CAD build for the part. Positions are in the model's coordinates, mm. Face numbers are marked on the shaded views. A direction names the side the tool comes from. Round coordinates to 2 decimals unless told otherwise and drop trailing zeros. Loops run counter-clockwise (first coordinate to the right, second up) from the corner with the lowest first, then second, coordinate; pieces in that order, holes last.
```python
from build123d import *

# Parameters (mm, degrees)
SKETCH1_W           = 86.36
SKETCH1_H           = 71.374
BOSS_EXTRUDE1_DEPTH = 39.624
FILLET1_R           = 2.54
CUT_EXTRUDE1_DEPTH  = 25.4
FILLET2_R           = 1.27
SKETCH4_W           = 49.53
SKETCH4_H           = 15.24
CUT_EXTRUDE2_DEPTH  = 50.8
SKETCH5_R           = 11.6205
BOSS_EXTRUDE2_DEPTH = 15.494
CUT_REVOLVE1_ANGLE  = 356


with BuildPart() as part:
    # Sketch1 → Boss-Extrude1 (new body)
    with BuildSketch(Plane(origin=(0, 0, 0), x_dir=(1, 0, 0), z_dir=(0, 1, 0))):
        with Locations((43.18, -35.687)):
            Rectangle(SKETCH1_W, SKETCH1_H)
    extrude(amount=BOSS_EXTRUDE1_DEPTH)

    # Fillet1
    fillet1_edges = [part.edges().sort_by_distance(p)[0] for p in [
        (0, 19.812, 0),
        (86.36, 19.812, 0),
        (86.36, 19.812, 71.374),
        (0, 19.812, 71.374),
    ]]
    fillet(fillet1_edges, radius=FILLET1_R)

    # Sketch2 → Cut-Extrude1 (cut)
    with BuildSketch(Plane.ZY):
        with BuildLine():
            Line((30.226, 33.02), (30.48, 33.02))
            ThreePointArc((30.48, 33.02), (31.737235857, 32.499235857), (32.258, 31.242))
            Line((32.258, 31.242), (32.258, 24.892))
            ThreePointArc((32.258, 24.892), (31.737235857, 23.634764143), (30.48, 23.114))
            Line((30.48, 23.114), (30.226, 23.114))
            ThreePointArc((30.226, 23.114), (28.968764143, 23.634764143), (28.448, 24.892))
            Line((28.448, 24.892), (28.448, 31.242))
            ThreePointArc((28.448, 31.242), (28.968764143, 32.499235857), (30.226, 33.02))
        make_face()
        with BuildLine():
            Line((41.148, 23.114), (40.894, 23.114))
            ThreePointArc((40.894, 23.114), (39.636764143, 23.634764143), (39.116, 24.892))
            Line((39.116, 24.892), (39.116, 31.242))
            ThreePointArc((39.116, 31.242), (39.636764143, 32.499235857), (40.894, 33.02))
            Line((40.894, 33.02), (41.148, 33.02))
            ThreePointArc((41.148, 33.02), (42.405235857, 32.499235857), (42.926, 31.242))
            Line((42.926, 31.242), (42.926, 24.892))
            ThreePointArc((42.926, 24.892), (42.405235857, 23.634764143), (41.148, 23.114))
        make_face()
    extrude(amount=-CUT_EXTRUDE1_DEPTH, mode=Mode.SUBTRACT)

    # Fillet2
    fillet2_edges = [part.edges().sort_by_distance(p)[0] for p in [
        (0, 23.634764143, 28.968764143),
        (0, 23.114, 30.353),
        (0, 23.634764143, 31.737235857),
        (0, 28.067, 32.258),
        (0, 32.499235857, 31.737235857),
        (0, 33.02, 30.353),
        (0, 32.499235857, 28.968764143),
        (0, 28.067, 28.448),
        (0, 23.634764143, 42.405235857),
        (0, 28.067, 42.926),
        (0, 32.499235857, 42.405235857),
        (0, 33.02, 41.021),
        (0, 32.499235857, 39.636764143),
        (0, 28.067, 39.116),
        (0, 23.634764143, 39.636764143),
        (0, 23.114, 41.021),
    ]]
    fillet(fillet2_edges, radius=FILLET2_R)

    # Sketch4 → Cut-Extrude2 (cut)
    with BuildSketch(Plane(origin=(86.36, 0, 0), x_dir=(0, 0, -1), z_dir=(1, 0, 0))):
        with Locations((-35.687, 9.0932)):
            Rectangle(SKETCH4_W, SKETCH4_H)
    extrude(amount=-CUT_EXTRUDE2_DEPTH, mode=Mode.SUBTRACT)

    # Sketch5 → Boss-Extrude2 (add)
    with BuildSketch(Plane(origin=(0, 39.624, 0), x_dir=(1, 0, 0), z_dir=(0, 1, 0))):
        with Locations(Location((28.448, -22.86, 0), (0, 0, 270))):
            Circle(SKETCH5_R)
    extrude(amount=BOSS_EXTRUDE2_DEPTH)

    # Sketch7 → Cut-Revolve1 (revolve, cut)
    with BuildSketch(Plane(origin=(0, 0, 22.86), x_dir=(-1, 0, 0), z_dir=(0, 0, -1))):
        Polygon((-16.8275, 42.164), (-20.3835, 43.727171461), (-21.3995, 55.118), (-16.8275, 55.118), align=None)
    revolve(axis=Axis((28.448, 55.118, 22.86), (0, 1, 0)), revolution_arc=CUT_REVOLVE1_ANGLE, mode=Mode.SUBTRACT)


solid = part.part
```
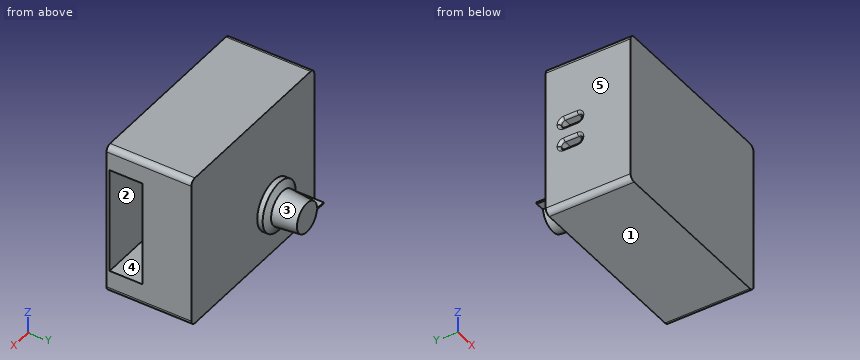
Item 1: Flat gauge pins, fed straight in: P1, Ø3, axis at y = 26.5, z = 40, coming from the -X side; P2, Ø25, axis at x = 59, z = 38, coming from the +Y side; P3, Ø3, axis at y = 27.5, z = 31.5, coming from the -X side. Where does each tip first touch, or does it go through?
Answers follow:
P1: stops at x = 0.18
P2: stops at y = 39.62
P3: stops at x = 0.11
Item 2: Cut at C-C, the plane x = 7.5. Give the cut face in (y, z), plus the area to 3 significant figures.
Answers follow:
outline: (0, 0) - (39.62, 0) - (39.62, 71.37) - (0, 71.37) - close; hole (23.11, 30.23) arc R1.78 ccw to (24.89, 28.45) - (31.24, 28.45) arc R1.78 ccw to (33.02, 30.23) - (33.02, 30.48) arc R1.78 ccw to (31.24, 32.26) - (24.89, 32.26) arc R1.78 ccw to (23.11, 30.48) - close; hole (23.11, 40.89) arc R1.78 ccw to (24.89, 39.12) - (31.24, 39.12) arc R1.78 ccw to (33.02, 40.89) - (33.02, 41.15) arc R1.78 ccw to (31.24, 42.93) - (24.89, 42.93) arc R1.78 ccw to (23.11, 41.15) - close
area: 2,760 mm2
Item 3: Probe line 1 (Z direction, x = 23, y = 31.5); line 2 (Z direction, x = 7, y = 30.5); line 3 (Y direction, x = 75, z = 40.5). List the from-to ranges inside material, lowest first.
Answers follow:
line 1: z = 0 to 28.47, 32.24 to 39.13, 42.91 to 71.37
line 2: z = 0 to 28.45, 32.26 to 39.12, 42.93 to 71.37
line 3: y = 0 to 1.47, 16.71 to 39.62
Item 4: Cut at D-D, the plane y = 29.5. Give the cut face in (x, z), plus the area to 3 significant figures.
Answers follow:
outline: (0, 2.54) arc R2.54 ccw to (2.54, 0) - (83.82, 0) arc R2.54 ccw to (86.36, 2.54) - (86.36, 68.83) arc R2.54 ccw to (83.82, 71.37) - (2.54, 71.37) arc R2.54 ccw to (0, 68.83) - (0, 44.2) arc R1.27 ccw to (1.27, 42.93) - (25.4, 42.93) - (25.4, 39.12) - (1.27, 39.12) arc R1.27 ccw to (0, 37.85) - (0, 33.53) arc R1.27 ccw to (1.27, 32.26) - (25.4, 32.26) - (25.4, 28.45) - (1.27, 28.45) arc R1.27 ccw to (0, 27.18) - close
area: 5,960 mm2
Item 5: Two-plate mould, pull along Y, no slides. Class the marked faces 3, 4 and 5: released by +Y, released by -Y, zero draft, split by the parting line, or undercut.
Answers follow:
face 3: released by +Y
face 4: undercut
face 5: zero draft
Item 6: Cut at A-A, the plane x = 73.5. Give the cut face in (y, z), plus the area to 3 significant figures.
Answers follow:
outline: (0, 0) - (39.62, 0) - (39.62, 71.37) - (0, 71.37) - close; hole (1.47, 10.92) - (16.71, 10.92) - (16.71, 60.45) - (1.47, 60.45) - close
area: 2,070 mm2
Item 7: 3-axis set-ups, long thin cutter, end or side, ignore diameter. For the marked faces 1 and 2: which of +Z, -Z, +X, -X, +Y, -Y reach the whole face in a straight line?
Answers follow:
face 1: -Z, +X, -X, +Y, -Y
face 2: +X
Item 8: Cut at B-B, the plane z = 51. Give the cut face in (x, y), plus the area to 3 significant figures.
Answers follow:
outline: (0, 0) - (86.36, 0) - (86.36, 1.47) - (35.56, 1.47) - (35.56, 16.71) - (86.36, 16.71) - (86.36, 39.62) - (0, 39.62) - close
area: 2,650 mm2
